For this review, take the finished solid that the model builds, in its own axes (mm). Face numbers are marked on the shaded views. A direction names the side the tool comes from. Give positions to 0.01 mm unless a question says otherwise; leave off trailing zeros. Order: outer loops, then holes, each group sorted by start corner. A loop starts at its lowest first (then second) coordinate and runs counter-clockwise, first axis right, second up. Notation, with made-up numbers: (13.25, 66.5) - (69.25, 66.5) arc R31 ccw to (69.25, 101.5) - close; hole circle Ø9 at (32, 27.25). An arc over 180 degrees is marked (long way). Put each result on its own line as item: value. Start each with the question number.
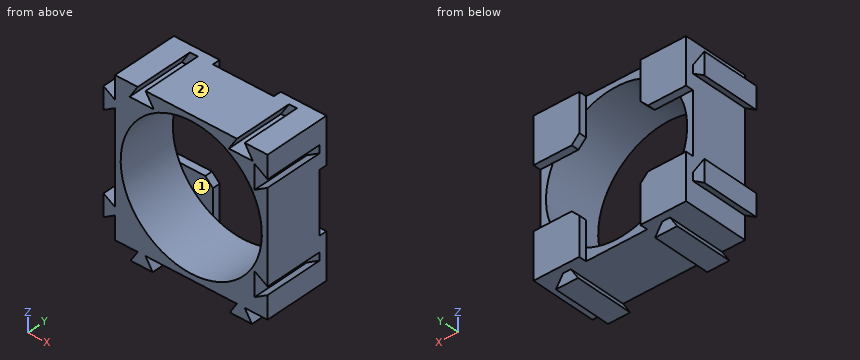
```python
from build123d import *

# Parameters (mm, degrees)
SKETCH1_R           = 9.25
BOSS_EXTRUDE1_DEPTH = 7.7
BOSS_EXTRUDE2_DEPTH = 1


with BuildPart() as part:
    # Sketch1 → Boss-Extrude1 (new body)
    with BuildSketch(Plane(origin=(0, 0, 0), x_dir=(1, 0, 0), z_dir=(0, 1, 0))):
        Polygon((-7.012695972, 10), (-7.95, 11.5), (-5.05, 11.5), (-5.987304028, 10), (5.987304028, 10), (5.05, 11.5), (7.95, 11.5), (7.012695972, 10), (10, 10), (10, 7.012695972), (8.3, 8.07497387), (8.3, 4.92502613), (10, 5.987304028), (10, -5.987304028), (8.3, -4.92502613), (8.3, -8.07497387), (10, -7.012695972), (10, -10), (7.012695972, -10), (8.07497387, -8.3), (4.92502613, -8.3), (5.987304028, -10), (-5.987304028, -10), (-4.92502613, -8.3), (-8.07497387, -8.3), (-7.012695972, -10), (-10, -10), (-10, -7.012695972), (-11.5, -7.95), (-11.5, -5.05), (-10, -5.987304028), (-10, 5.987304028), (-11.5, 5.05), (-11.5, 7.95), (-10, 7.012695972), (-10, 10), align=None)
        with Locations(Location((0, 0, 0), (0, 0, 90))):
            Circle(SKETCH1_R, mode=Mode.SUBTRACT)
    extrude(amount=BOSS_EXTRUDE1_DEPTH)

    # Sketch2 → Boss-Extrude2 (add)
    with BuildSketch(Plane(origin=(0, 7.7, 0), x_dir=(1, 0, 0), z_dir=(0, 1, 0))):
        Polygon((-5, -4), (-4, -5), (-4, -10), (-10, -10), (-10, -4), align=None)
        Polygon((-4, 10), (-4, 5), (-5, 4), (-10, 4), (-10, 10), align=None)
        Polygon((10, 4), (5, 4), (4, 5), (4, 10), (10, 10), align=None)
        Polygon((4, -10), (4, -5), (5, -4), (10, -4), (10, -10), align=None)
    extrude(amount=BOSS_EXTRUDE2_DEPTH)


solid = part.part
```
1. Add section A-A, the plane x = 0. Give the boundary of the cut face in (y, z).
2. Clearance check with flat-ended pins moving along their axes: pin 1 (1.8 mm diameter, centred on x = 1, z = -9.5, fed in from +Y); pin 2 (0.5 mm diameter, centred on x = -7, z = 9, fed in from -Y); pin 3 (4 mm diameter, centred on y = 4.5, z = -0.5, fed in from -X). State where each tip first meets the part, or that it passes through.
3. Add section B-B, the plane z = 0. Give the boundary of the cut face in (x, y), then the cut area to 4 significant figures.
4. Add section C-C, the plane z = -5.5. Give the boundary of the cut face in (x, y), then the cut area to 3 significant figures.
5. Wall thickness on line 1 (X direction, y = 4.25, z = 5.25); line 2 (X direction, y = 3.75, z = 0); line 3 (X direction, y = 2, z = 4.5): over which ranges is each line inside the solid? List them lowest first. Write a range as from..to.
6. Tool access review of the marked faces 1 and 2: name each direction out of +Z, -Z, +X, -X, +Y, -Y from which nothing blocks a thin tool from reaching the whole face with its end or side.
Found:
1. outline: (0, -10) - (7.7, -10) - (7.7, -9.25) - (0, -9.25) - close; (0, 9.25) - (7.7, 9.25) - (7.7, 10) - (0, 10) - close
2. pin 1: stops at y = 7.7
2. pin 2: stops at y = 7.7
2. pin 3: stops at x = -10
3. outline: (-10, 0) - (-9.25, 0) - (-9.25, 7.7) - (-10, 7.7) - close; (9.25, 0) - (10, 0) - (10, 7.7) - (9.25, 7.7) - close
3. area: 11.55 mm^2
4. outline: (-11.5, 0) - (-10.78, 0) - (-10.78, 7.7) - (-11.5, 7.7) - close; (-10, 0) - (-7.44, 0) - (-7.44, 7.7) - (-4, 7.7) - (-4, 8.7) - (-10, 8.7) - close; (4, 7.7) - (7.44, 7.7) - (7.44, 0) - (8.3, 0) - (8.3, 7.7) - (9.22, 7.7) - (9.22, 0) - (10, 0) - (10, 8.7) - (4, 8.7) - close
4. area: 49.9 mm^2
5. line 1: x = -11.5..-11.18, -10..-7.62, 7.62..8.3, 8.82..10
5. line 2: x = -10..-9.25, 9.25..10
5. line 3: x = -10..-8.08, 8.08..10
6. face 1: -Y
6. face 2: +Z, +X, -X, +Y, -Y
